```python
from build123d import *

# Parameters (mm, degrees)
SKETCH1_W           = 138
SKETCH1_H           = 46
BOSS_EXTRUDE1_DEPTH = 19.5
SKETCH2_W           = 6
SKETCH2_H           = 12
BOSS_EXTRUDE2_DEPTH = 3
CHAMFER1_SIZE       = 1


with BuildPart() as part:
    # Sketch1 → Boss-Extrude1 (new body, symmetric)
    with BuildSketch(Plane.XY):
        Rectangle(SKETCH1_W, SKETCH1_H)
    extrude(amount=BOSS_EXTRUDE1_DEPTH, both=True)

    # Sketch2 → Boss-Extrude2 (add, symmetric)
    with BuildSketch(Plane(origin=(69, 0, 0), x_dir=(0, 0, -1), z_dir=(1, 0, 0))):
        with Locations((-16.5, 0)):
            Rectangle(SKETCH2_W, SKETCH2_H)
    extrude(amount=BOSS_EXTRUDE2_DEPTH, both=True)

    # Chamfer1
    chamfer1_edges = [part.edges().sort_by_distance(p)[0] for p in [
        (-69, 0, 19.5),
        (0, -23, 19.5),
        (69, 14.5, 19.5),
        (69, 0, 13.5),
        (70.5, 6, 19.5),
        (70.5, -6, 13.5),
        (70.5, -6, 19.5),
        (69, -6, 16.5),
        (70.5, 6, 13.5),
        (69, 6, 16.5),
        (72, 0, 19.5),
        (72, -6, 16.5),
        (72, 0, 13.5),
        (72, 6, 16.5),
        (69, -14.5, 19.5),
        (0, -23, -19.5),
        (-69, 0, -19.5),
        (0, 23, -19.5),
        (69, 0, -19.5),
        (69, -23, 0),
        (-69, -23, 0),
        (-69, 23, 0),
        (69, 23, 0),
        (0, 23, 19.5),
    ]]
    chamfer(chamfer1_edges, length=CHAMFER1_SIZE)


solid = part.part
```
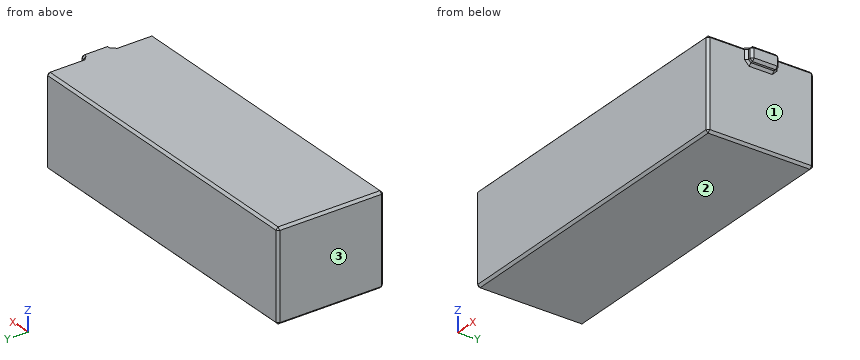
Geometry: final body of the model. Coordinates: model frame, mm. Face numbers are marked on the shaded views. Round coordinates to 2 decimals unless told otherwise and drop trailing zeros. Order: outer loops, then holes, each group sorted by start corner. A loop starts at its lowest first (then second) coordinate and runs counter-clockwise, first axis right, second up. Notation, with made-up numbers: (-12.75, 59.25) - (16.25, 59.25) arc R26 cw to (16.25, 89.25) - close; hole circle Ø8 at (31.25, 61). An arc over 180 degrees is marked (long way). Write item = value, one per line. Start each with the question number.
Q1. Cut plane A-A on z = -9.5. Return the cut outline in (x, y), and give its area (3 significant figures).
Q2. Cut plane B-B on y = 13.5. Return the cut outline in (x, z).
Q3. Ray query, line 1 (X direction, y = -7, z = -4). Return the intervals inside material, ascending. Write a range as from..to.
Q4. Pull-direction query (X, two-part tool) for the marked faces 1, 2 and 3; classes: +X half, -X half, draft (parallel to the pull), parting line (faces both ways), or undercut.
Q5. Pin query (flat end, axial travel): pin 1 (0.5 mm diameter, centred on x = 70.5, z = 17.5, fed in from +Y); pin 2 (0.5 mm diameter, centred on x = 70.5, z = 15.5, fed in from -Y); pin 3 (0.5 mm diameter, centred on x = 70.5, y = -2.5, fed in from -Z). Return the tip coordinate at first contact, or that it passes through.
Outcome:
q1.outline = (-69, -22) - (-68, -23) - (68, -23) - (69, -22) - (69, 22) - (68, 23) - (-68, 23) - (-69, 22) - close
q1.area = 6,350 mm^2
q2.outline = (-69, -18.5) - (-68, -19.5) - (68, -19.5) - (69, -18.5) - (69, 18.5) - (68, 19.5) - (-68, 19.5) - (-69, 18.5) - close
q3.line_1 = -69..69
q4.face_1 = +X half
q4.face_2 = draft
q4.face_3 = -X half
q5.pin_1 = 6
q5.pin_2 = -6
q5.pin_3 = 13.5
